Work out the finished part from the listing and answer in its coordinate system (mm). A direction names the side the tool comes from. Give positions to 0.01 mm unless a question says otherwise; leave off trailing zeros. Write each loop counter-clockwise with the first axis right and the second up, starting at its lowest first coordinate (ties: lowest second). Pieces come first, ordered by that corner, then holes. Notation, with made-up numbers: (35, -7.5) -> (72, -7.5) arc R32 cw to (72, 20.5) -> close; hole circle Ø1 at (-25.75, 42.25). An arc over 180 degrees is marked (long way). Write item = value, one per line. Start each with the question number.
from build123d import *

# Parameters (mm, degrees)
F1_DEPTH = 2


# Not quite as in the source:
# - a feature names something its author has since deleted; it is built from what else it names


with BuildPart() as f1:
    # F0 (on Top) → F1 (new body)
    with BuildSketch(Plane.XY):
        with BuildLine():
            Line((-17.7180729806, 0), (-13.3472634479, 0))
            ThreePointArc((-13.3472634479, 0), (-5.6771986993, 10.9915241569), (0, 23.1328960508))
            ThreePointArc((0, 23.1328960508), (-11.5247073045, 55.6975197064), (-37.5854000449, 78.3715993166))
            ThreePointArc((-37.5854000449, 78.3715993166), (-36.1278357664, 114.3054992712), (-12.5523087913, 141.4636322597))
            ThreePointArc((-12.5523087913, 141.4636322597), (19.6930692126, 127.5307837734), (42.0421807398, 100.4308597236))
            ThreePointArc((42.0421807398, 100.4308597236), (65.4226402571, 72.3273330377), (99.6574273635, 59.5041723042))
            Line((99.6574273635, 59.5041723042), (97.2733384301, 51.1598982899))
            ThreePointArc((97.2733384301, 51.1598982899), (116.6670679291, 50.9395271005), (134.6239036251, 43.610314378))
            Line((134.6239036251, 43.610314378), (135.8159518172, 49.5705106347))
            Line((135.8159518172, 49.5705106347), (103.4726053476, 70.4246684909))
            ThreePointArc((103.4726053476, 70.4246684909), (63.5065429383, 109.2866549818), (24.0146897469, 148.6304431832))
            Line((24.0146897469, 148.6304431832), (-12.1552264318, 148.3045816422))
            Line((-12.1552264318, 148.3045816422), (-29.2411223054, 148.3045816422))
            Line((-29.2411223054, 148.3045816422), (-73.3465850353, 147.9072272778))
            ThreePointArc((-73.3465850353, 147.9072272778), (-53.9798913788, 82.6367857077), (-12.9499193281, 28.30594033))
            Line((-12.9499193281, 28.30594033), (-17.7180729806, 0))
        make_face()
    extrude(amount=F1_DEPTH)


solid = f1.part
(1) For faces 4 (the flat face through (119.87, 59.85, 0.99)), 5 (the cylindrical face through (-11.25, 55.29, 0.99)), determine the directions among +Z, -Z, +X, -X, +Y, -Y from which every point of the face is accessible in a straight line to the end or side of a thin tool.
(2) Each of these flat-tipped pins is pushed along its axis until it touches: pin 1 (1 mm diameter, centred on y = 76, z = 1, fed in from +X); pin 2 (0.6 mm diameter, centred on x = -18, z = 0.5, fed in from +Y). Where does it stop, or does it pass through?
(3) A cutting plane is placed at C-C, the plane z = 0.4. Write down the section's boundary in (x, y), then the cut area to 3 significant figures.
(4) A cutting plane is placed at B-B, the plane x = -6.5. Write down the section's boundary in (y, z).
(5) A cutting plane is placed at D-D, the plane x = 119. Write down the section's boundary in (y, z).
(6) Determine the mould class of faces 1 (the flat face through (-15.3, 14.35, 0.99)), 2 (the cylindrical face through (116.399, 50.993, 0.986)), 3 (the flat face through (31, 119, 0)) for opening direction X: pulls with the +X half, pulls with the -X half, needs draft (parallel to the pull), parting line crosses it, or undercut.
(7) A cutting plane is placed at A-A, the plane y = 107. Write down the section's boundary in (x, z), then the cut area to 3 significant figures.
(8) Find the intervals of material crossed by line 1 along X through (y, z) = (120.5, 1.85); line 2 along X through (y, z) = (134, 0.9); line 3 along Y through (x, z) = (-27.5, 0.9), in increasing order.
Results list:
q1.face_4 = +Z, -Z, +X, +Y
q1.face_5 = +Z, -Z
q2.pin_1 = 98.2
q2.pin_2 = 148.3
q3.outline = (-73.35, 147.91) arc R191 ccw to (-12.95, 28.31) -> (-17.72, 0) -> (-13.35, 0) arc R78.08 ccw to (0, 23.13) arc R67.87 ccw to (-37.59, 78.37) arc R54.35 cw to (-12.55, 141.46) arc R74.91 cw to (42.04, 100.43) arc R71.3 ccw to (99.66, 59.5) -> (97.27, 51.16) arc R51.87 cw to (134.62, 43.61) -> (135.82, 49.57) -> (103.47, 70.42) arc R4596.8 cw to (24.01, 148.63) -> (-12.16, 148.3) -> (-29.24, 148.3) -> close
q3.area = 6,830 mm²
q4.outline = (9.6, 0) -> (46.99, 0) -> (46.99, 2) -> (9.6, 2) -> close; (140.16, 0) -> (148.36, 0) -> (148.36, 2) -> (140.16, 2) -> close
q5.outline = (50.41, 0) -> (60.41, 0) -> (60.41, 2) -> (50.41, 2) -> close
q6.face_1 = pulls with the -X half
q6.face_2 = undercut
q6.face_3 = needs draft
q7.outline = (-64.23, 0) -> (-38.45, 0) -> (-38.45, 2) -> (-64.23, 2) -> close; (38.43, 0) -> (65.83, 0) -> (65.83, 2) -> (38.43, 2) -> close
q7.area = 106 mm²
q8.line_1 = -68.29 to -33.21, 27.77 to 52.15
q8.line_2 = -71.3 to -22.69, 9.46 to 38.59
q8.line_3 = 43.27 to 72.25, 128.89 to 148.3
